Geometry: final body of the model. Coordinates: model frame, mm. Coordinates: 2 decimals unless noted, no trailing zeros. Write each loop counter-clockwise with the first axis right and the second up, starting at its lowest first coordinate (ties: lowest second). Pieces come first, ordered by that corner, then holes. Notation, with made-up numbers: (-14.5, 65) - (29.5, 65) arc R16 ccw to (29.5, 83) - close; hole circle Ø6 at (-22, 65). An arc over 180 degrees is marked (long way). Answer as a JSON object with one key per item and string values. Group by question number.
Item 1: Line query: line 1 along X through (y, z) = (302.75, -186.5); line 2 along X through (y, z) = (303, -250) (3 decimals); line 3 along Z through (x, y) = (900, 304.5) (3 decimals). Output: solid intervals per line, ascending. Write a range as from..to.
Item 2: Section B-B on y = 303.75. Return loops of the section in (x, z) (3 decimals), and give its area (3 significant figures).
Item 3: Section A-A on x = 900. Return loops of the section in (y, z) (3 decimals).
Item 4: First-contact query: pin 1 Ø21.5 at (x, z) = (900, -250) entering from +Y; pin 2 Ø6.5 at (x, y) = (792, 304) entering from +Z. Flat tips, straight axial feed; report the tip coordinate or a pass-through.
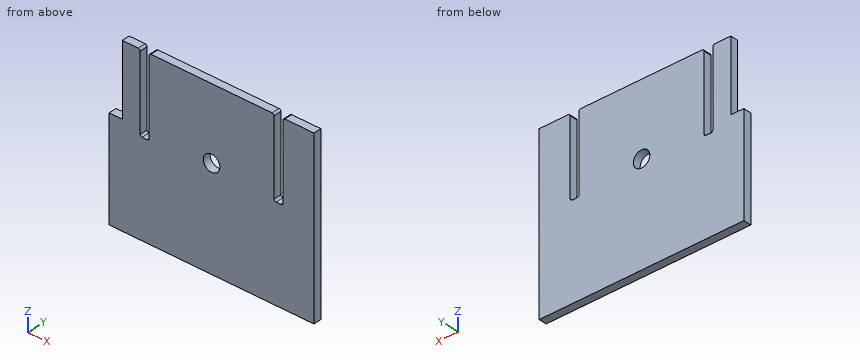
```python
from build123d import *

# Parameters (mm, degrees)
BOSS_EXTRUDE1_DEPTH  = 12.7
CAVITY1_START        = 298.45
CAVITY1_OUTLINE_R    = 12.7
CAVITY1_DEPTH        = 12.7
CAVITY1_START_2      = 720.91620239
CAVITY1_2_DEPTH      = 22.43918751
SKETCH2_W            = 21.068746236
SKETCH2_H            = 115.32536453
CUT_EXTRUDE1_DEPTH   = 1143.349273427
MOVE_FACE_SLOTS_BY   = 0.762
MOVE_FACE_SLOTS_2_BY = 0.762
MOVE_FACE_SLOTS_3_BY = 0.762
MOVE_FACE_SLOTS_4_BY = 0.762
MOVE_FACE_SLOTS_5_BY = 0.762
MOVE_FACE_SLOTS_6_BY = 0.762
MOVE_FACE_HOLES_BY   = 0.635
SLOT_FILLETS_R       = 3.175


# Read off the part's stored shape, not the designer's step: Cavity1
with BuildPart() as part:
    # Sketch1 → Boss-Extrude1 (new body)
    with BuildSketch(Plane(origin=(0, 298.45, 0), x_dir=(-1, 0, 0), z_dir=(0, -1, 0))):
        Polygon((-798.4, 260.35), (-798.4, 133.35), (-1001.6, 133.35), (-1001.6, 260.35), (-1014.3, 260.35), (-1014.3, 133.35), (-1065.1, 133.35), (-1065.1, 412.75), (-1014.3, 412.75), (-1001.6, 412.75), (-798.4, 412.75), (-785.7, 412.75), (-734.9, 412.75), (-734.9, 133.35), (-785.7, 133.35), (-785.7, 260.35), align=None)
    extrude(amount=-BOSS_EXTRUDE1_DEPTH)

    # Cavity1 outline → Cavity1 (cut)
    with BuildSketch(Plane(origin=(0, 0, 0), x_dir=(1, 0, 0), z_dir=(0, 1, 0)).offset(CAVITY1_START)):
        with Locations((900, 250)):
            Circle(CAVITY1_OUTLINE_R)
    extrude(amount=CAVITY1_DEPTH, mode=Mode.SUBTRACT)

    # Cavity1 2 outline → Cavity1 2 (cut)
    with BuildSketch(Plane(origin=(0, 0, 0), x_dir=(0.7149295353100682, -0.6987525164445135, -0.024913456279483565), z_dir=(0.6991965099607762, 0.7144755512387232, 0.02547404837855681)).offset(CAVITY1_START_2)):
        with BuildLine():
            ThreePointArc((313.444242413, 230.081087528), (327.146171675, 242.424687318), (314.076314529, 255.435688643))
            Line((314.076314529, 255.435688643), (312, 255.374549574))
            Line((312, 255.374549574), (312, 230.195835843))
            Line((312, 230.195835843), (313.444242413, 230.081087528))
        make_face()
    extrude(amount=CAVITY1_2_DEPTH, mode=Mode.SUBTRACT)

    # Sketch2 → Cut-Extrude1 (cut, through all)
    with BuildSketch(Plane(origin=(0, 311.15, 0), x_dir=(1, 0, 0), z_dir=(0, 1, 0))):
        with Locations((745.434373118, 191.012682265)):
            Rectangle(SKETCH2_W, SKETCH2_H)
    extrude(amount=-CUT_EXTRUDE1_DEPTH, mode=Mode.SUBTRACT)

    # Move Face Slots: a face moved inward by 0.762
    extrude(part.faces().sort_by_distance((1001.6, 304.8, -196.85))[0], amount=MOVE_FACE_SLOTS_BY, dir=(-1, 0, 0), mode=Mode.SUBTRACT)

    # Move Face Slots 2: a face moved inward by 0.762
    extrude(part.faces().sort_by_distance((785.7, 304.8, -196.85))[0], amount=MOVE_FACE_SLOTS_2_BY, dir=(-1, 0, 0), mode=Mode.SUBTRACT)

    # Move Face Slots 3: a face moved inward by 0.762
    extrude(part.faces().sort_by_distance((1014.3, 304.8, -196.85))[0], amount=MOVE_FACE_SLOTS_3_BY, dir=(1, 0, 0), mode=Mode.SUBTRACT)

    # Move Face Slots 4: a face moved inward by 0.762
    extrude(part.faces().sort_by_distance((1007.95, 304.8, -260.35))[0], amount=MOVE_FACE_SLOTS_4_BY, dir=(0, 0, -1), mode=Mode.SUBTRACT)

    # Move Face Slots 5: a face moved inward by 0.762
    extrude(part.faces().sort_by_distance((798.4, 304.8, -196.85))[0], amount=MOVE_FACE_SLOTS_5_BY, dir=(1, 0, 0), mode=Mode.SUBTRACT)

    # Move Face Slots 6: a face moved inward by 0.762
    extrude(part.faces().sort_by_distance((792.05, 304.8, -260.35))[0], amount=MOVE_FACE_SLOTS_6_BY, dir=(0, 0, -1), mode=Mode.SUBTRACT)

    # Move Face Holes: a curved face moved inward by 0.635
    add(Solid.thicken(part.faces().sort_by_distance((887.3, 304.8, -250))[0], -MOVE_FACE_HOLES_BY), mode=Mode.SUBTRACT)

    # Slot Fillets
    slot_fillets_edges = [part.edges().sort_by_distance(p)[0] for p in [
        (799.162, 304.8, -261.112),
        (799.162, 304.8, -133.35),
        (1000.838, 304.8, -133.35),
        (1000.838, 304.8, -261.112),
        (1015.062, 304.8, -261.112),
        (1015.062, 304.8, -133.35),
        (784.938, 304.8, -133.35),
        (784.938, 304.8, -261.112),
    ]]
    fillet(slot_fillets_edges, radius=SLOT_FILLETS_R)


solid = part.part
```
Checks:
{
 "1": {"line 1": "755.97..784.94, 799.16..1000.84, 1015.06..1065.1", "line 2": "734.9..784.938, 799.162..886.665, 913.335..1000.838, 1015.062..1065.1", "line 3": "-412.75..-263.335, -236.665..-133.35"},
 "2": {"outline": "(734.9, -412.75) - (1065.1, -412.75) - (1065.1, -133.35) - (1018.237, -133.35) arc R3.175 ccw to (1015.062, -136.525) - (1015.062, -257.937) arc R3.175 cw to (1011.887, -261.112) - (1004.013, -261.112) arc R3.175 cw to (1000.838, -257.937) - (1000.838, -136.525) arc R3.175 ccw to (997.663, -133.35) - (802.337, -133.35) arc R3.175 ccw to (799.162, -136.525) - (799.162, -257.937) arc R3.175 cw to (795.987, -261.112) - (788.113, -261.112) arc R3.175 cw to (784.938, -257.937) - (784.938, -136.525) arc R3.175 ccw to (781.763, -133.35) - (755.969, -133.35) - (755.969, -248.675) - (734.9, -248.675) - close; hole circle Ø26.67 at (900, -250)", "area": "85,600 mm^2"},
 "3": {"outline": "(298.45, -412.75) - (311.15, -412.75) - (311.15, -263.335) - (298.45, -263.335) - close; (298.45, -236.665) - (311.15, -236.665) - (311.15, -133.35) - (298.45, -133.35) - close"},
 "4": {"pin 1": "through", "pin 2": "z = -261.11"}
}
